Could you check a few things on this model? Use its own coordinates, in mm. A direction names the side the tool comes from. Give positions to 0.01 mm unless a question says otherwise; leave off trailing zeros. Write each loop counter-clockwise with the first axis right and the second up, starting at its lowest first coordinate (ties: lowest second). Pieces come first, ordered by that corner, then holes. Notation, with made-up numbers: (50, 22) - (83, 22) arc R34 ccw to (83, 53) - close; hole circle Ø4 at (-2.5, 47). An arc over 180 degrees is marked (long way). Write item = value, one per line.
from build123d import *

# Parameters (mm, degrees)
SKETCH_R     = 2.8
PAD_DEPTH    = 3
SKETCH001_R  = 1.45
PAD001_DEPTH = 6
POCKET_DEPTH = 2
CHAMFER_SIZE = 0.25


with BuildPart() as part:
    # Sketch → Pad (new body)
    with BuildSketch(Plane.XY):
        Circle(SKETCH_R)
    extrude(amount=PAD_DEPTH)

    # Sketch001 (on Face3 of Pad) → Pad001 (join)
    with BuildSketch(Plane.XY.offset(3)):
        Circle(SKETCH001_R)
    extrude(amount=PAD001_DEPTH)

    # Sketch002 (on Face2 of Pad001) → Pocket (cut)
    with BuildSketch(Plane(origin=(0, 0, 0), x_dir=(1, 0, 0), z_dir=(0, 0, -1))):
        Polygon((1.259542, 0.814588), (-0.075682, 1.49809), (-1.335225, 0.683502), (-1.259542, -0.814588), (0.075682, -1.49809), (1.335225, -0.683502), align=None)
    extrude(amount=-POCKET_DEPTH, mode=Mode.SUBTRACT)

    # Chamfer
    chamfer_edges = [part.edges().sort_by_distance(p)[0] for p in [
        (-2.8, 0, 3),
        (-2.8, 0, 0),
        (1.297384, -0.065543, 0),
        (0.705454, 1.090796, 0),
        (-0.59193, 1.156339, 0),
        (-1.297384, 0.065543, 0),
        (-0.705454, -1.090796, 0),
        (0.59193, -1.156339, 0),
        (-1.45, 0, 9),
    ]]
    chamfer(chamfer_edges, length=CHAMFER_SIZE)


solid = part.part
1. I need wall thicknesses on line 1 (Z direction, x = 0.8, y = -2.35); line 2 (Y direction, x = -0.3, z = 1.75); line 3 (X direction, y = 0.85, z = 1.5). Which ranges of each line are inside material? Lowest first, please.
Filled sheet:
line_1 = 0 to 3
line_2 = -2.78 to -1.35, 1.31 to 2.78
line_3 = -2.67 to -1.19, 1.08 to 2.67
2. For pin 1 (2 mm diameter, centred on y = 1, z = 8, fed in from +X); pin 2 (1 mm diameter, centred on x = 1.5, z = 6.5, fed in from +Y); pin 3 (2 mm diameter, centred on x = 1, z = 8, fed in from +Y), each with a flat end and sliding along its axis, tell me the tip position at first contact or that it passes through.
Filled sheet:
pin_1 = 1.45
pin_2 = 1.05
pin_3 = 1.45
3. Thinking about a two-plate mould opening in X: for faces 1 (the face through (-2.8, 0.1, 1.5)), 2 (the face through (0, 0, 2)), 3 (the face through (0, -2, 3)), which applies, pulls with the +X half, pulls with the -X half, needs draft (parallel to the pull), parting line crosses it, or undercut?
Filled sheet:
face_1 = parting line crosses it
face_2 = undercut
face_3 = needs draft
4. Which directions (+Z, -Z, +X, -X, +Y, -Y) give clear straight access to the entire face, cutting with the end or side of a thin tool? Please do faces 4 (the face through (-1.45, 0.06, 5.83)), 5 (the face through (0.659, -1.26, 0.127)), 6 (the face through (2, 0, 0)).
Filled sheet:
face_4 = +Z
face_5 = -Z
face_6 = -Z, +X, -X, +Y, -Y
5. If we section it at B-B, the plane z = 3.75: Please give me the cut outline in (x, y).
Filled sheet:
outline = circle Ø2.9 at (0, 0)
6. If we section it at A-A, the plane y = 0: Please give me the cut outline in (x, z), and give its area (3 significant figures).
Filled sheet:
outline = (-2.8, 0.25) - (-2.55, 0) - (-1.55, 0) - (-1.3, 0.25) - (-1.3, 2) - (1.3, 2) - (1.3, 0.25) - (1.55, 0) - (2.55, 0) - (2.8, 0.25) - (2.8, 2.75) - (2.55, 3) - (1.45, 3) - (1.45, 8.75) - (1.2, 9) - (-1.2, 9) - (-1.45, 8.75) - (-1.45, 3) - (-2.55, 3) - (-2.8, 2.75) - close
area = 28.7 mm2
